Drawing for the job (mm, zero at the part's lowest x, y, z). A direction names the side the tool comes from. Coordinates: 2 decimals unless noted, no trailing zeros. Loops run counter-clockwise (first coordinate to the right, second up) from the corner with the lowest first, then second, coordinate; pieces in that order, holes last.
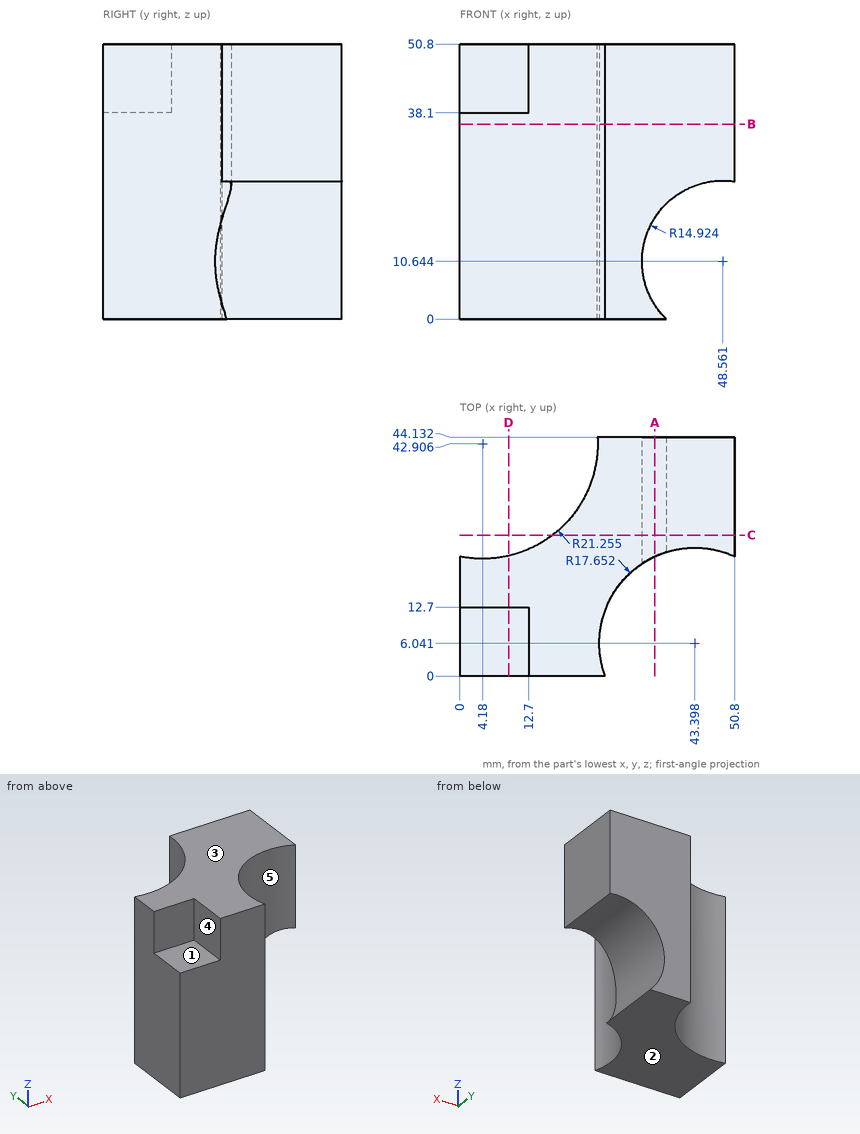
Q1. Saw through at C-C (y = 26). List the corners of the cut face in (x, z) (1 decimal).
Q2. Saw through at B-B (z = 36). List the corners of the cut face in (x, y) (1 decimal).
Q3. Saw through at A-A (x = 36). List the corners of the cut face in (y, z) (1 decimal), plus the area to 3 significant figures.
Q4. Mould opens along X. For the marked faces 3, 4 and 5 say: released by +X, released by -X, zero draft, split by the parting line, or undercut.
Q5. Drop flat-ended pins along their axis: P1, Ø6.5, axis at x = 6, z = 44, coming from the -Y side; P2, Ø6.5, axis at x = 7.5, y = 7, coming from the +Z side; P3, Ø4, axis at x = 31.5, z = 20.5, coming from the -Y side (1 decimal). Give the stop position or say it passes through.
Q6. Tool access for the marked faces 1 and 2: list every direction of +Z, -Z, +X, -X, +Y, -Y with a clear straight run to the whole face (end or side of a thin tool).
Q7. Saw through at D-D (x = 9). List the corners of the cut face in (y, z) (1 decimal).
Q8. Probe line 1 (Y direction, x = 4.5, z = 48); line 2 (Z direction, x = 46.5, y = 41) (1 decimal); line 3 (X direction, y = 10, z = 16.5) (1 decimal). List the from-to ranges inside material, lowest first.
Checked values:
1. outline: (17.1, 0) - (38.1, 0) arc R14.9 cw to (50.8, 25.4) - (50.8, 50.8) - (17.1, 50.8) - close
2. outline: (0, 0) - (26.8, 0) arc R17.7 cw to (50.8, 22.1) - (50.8, 44.1) - (25.4, 44.1) arc R21.3 cw to (0, 22.1) - close
3. outline: (22.1, 0) - (44.1, 0) - (44.1, 2.6) - (22.1, 2.6) - close; (22.1, 18.7) - (44.1, 18.7) - (44.1, 50.8) - (22.1, 50.8) - close
3. area: 765 mm2
4. face 3: zero draft
4. face 4: released by -X
4. face 5: undercut
5. P1: stops at y = 12.7
5. P2: stops at z = 38.1
5. P3: stops at y = 16.9
6. face 1: +Z, -X, -Y
6. face 2: -Z, +X, -X, +Y, -Y
7. outline: (0, 0) - (22.2, 0) - (22.2, 50.8) - (12.7, 50.8) - (12.7, 38.1) - (0, 38.1) - close
8. line 1: y = 12.7 to 21.65
8. line 2: z = 25.4 to 50.8
8. line 3: x = 0 to 26.2
